Work out the finished part from the listing and answer in its coordinate system (mm). Face numbers are marked on the shaded views. A direction names the side the tool comes from. Coordinates: 2 decimals unless noted, no trailing zeros. Order: outer loops, then holes, each group sorted by start corner. A loop starts at its lowest first (then second) coordinate and runs counter-clockwise, first axis right, second up. Notation, with made-up numbers: M 77,13 L 132,13 A24 ccw 132,38 Z; hole C 19.25,69.5 d3. An arc over 180 degrees is marked long. Use a Markdown table: item, result. Add a question column.
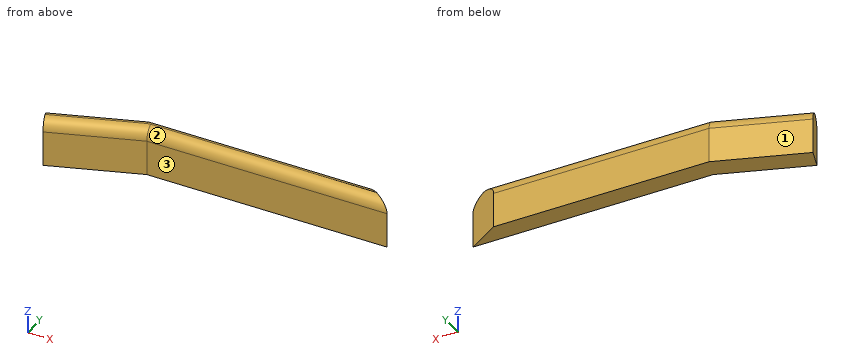
from build123d import *

# Parameters (mm, degrees)
SKETCH_1_W          = 20
SKETCH_1_H          = 4
EXTRUDE_1_DEPTH     = 1.75
EXTRUDE_2_DEPTH     = 4
EXTRUDE_3_DEPTH     = 4
CUT_EXTRUDE_1_DEPTH = 24.299797316
FILLET_4_R          = 1


with BuildPart() as part:
    # 草图1 → 凸台-拉伸1 (new body)
    with BuildSketch(Plane(origin=(0, 0, 0), x_dir=(1, 0, 0), z_dir=(0, 1, 0))):
        with Locations((10, -2)):
            Rectangle(SKETCH_1_W, SKETCH_1_H)
    extrude(amount=EXTRUDE_1_DEPTH)

    # 草图6 → 凸台-拉伸2 (add)
    with BuildSketch(Plane.XY.offset(4)):
        with BuildLine():
            Line((20, 0), (22.790216698, 0))
            ThreePointArc((22.790216698, 0), (21.391749441, 0.869644524), (20, 1.75))
            Line((20, 1.75), (20, 0))
        make_face()
    extrude(amount=-EXTRUDE_2_DEPTH)

    # 草图7 → 凸台-拉伸3 (add)
    with BuildSketch(Plane(origin=(0, 0, 0), x_dir=(-1, 0, 0), z_dir=(0, 0, -1))):
        Polygon((5.699396556, -2.736161147), (-1.818144411, 0), (-1.181196501, 1.75), (6.336344466, -0.986161147), align=None)
    extrude(amount=-EXTRUDE_3_DEPTH)

    # 草图8 → 切除-拉伸1 (cut, through all)
    with BuildSketch(Plane.XY.offset(4)):
        Polygon((1.181196501, 1.75), (-6.336344466, -0.986161147), (0, 1.75), align=None)
    extrude(amount=-CUT_EXTRUDE_1_DEPTH, mode=Mode.SUBTRACT)

    # 圆角4
    # the kernel refuses this fillet: 1 mm, written as the material it takes off along each edge
    with BuildSketch(Plane(origin=(-8.048628108, -3.591211505, 4), x_dir=(-0.3420201433256633, 0.9396926207859104, 0), z_dir=(0.9396926207859104, 0.3420201433256633, 0))) as fillet_4_piece_1_section:
        with BuildLine():
            CenterArc((FILLET_4_R, -FILLET_4_R), FILLET_4_R, 90, 90)
            Line((0, -FILLET_4_R), (0, 0))
            Line((0, 0), (FILLET_4_R, 0))
        make_face()
    fillet_4_piece_1 = extrude(amount=13, mode=Mode.PRIVATE)
    fillet_4_piece_1 = fillet_4_piece_1 - Plane(origin=(-8.048628108, 1, 3), x_dir=(0, 0, 1), z_dir=(-1, 0, 0)) * Cylinder(1, 31, mode=Mode.PRIVATE)
    add(fillet_4_piece_1, mode=Mode.SUBTRACT)
    with BuildSketch(Plane(origin=(-0.681855589, 0, 4), x_dir=(0, 1, 0), z_dir=(1, 0, 0))) as fillet_4_piece_2_section:
        with BuildLine():
            CenterArc((FILLET_4_R, -FILLET_4_R), FILLET_4_R, 90, 90)
            Line((0, -FILLET_4_R), (0, 0))
            Line((0, 0), (FILLET_4_R, 0))
        make_face()
    fillet_4_piece_2 = extrude(amount=25.972072288, mode=Mode.PRIVATE)
    fillet_4_piece_2 = fillet_4_piece_2 - Plane(origin=(-0.731431287, 0.136208109, 3), x_dir=(0, 0, 1), z_dir=(-0.9396926207859104, -0.3420201433256633, 0)) * Cylinder(1, 56, mode=Mode.PRIVATE)
    add(fillet_4_piece_2, mode=Mode.SUBTRACT)
    with BuildSketch(Plane(origin=(5.174890139, 3.203585609, 4), x_dir=(0.34202014332566305, -0.9396926207859104, 0), z_dir=(-0.9396926207859105, -0.3420201433256631, 0))) as fillet_4_piece_3:
        with BuildLine():
            CenterArc((FILLET_4_R, -FILLET_4_R), FILLET_4_R, 90, 90)
            Line((0, -FILLET_4_R), (0, 0))
            Line((0, 0), (FILLET_4_R, 0))
        make_face()
    extrude(amount=14.75, mode=Mode.SUBTRACT)
    with BuildSketch(Plane(origin=(22.5, 1.75, 4), x_dir=(0, -1, 0), z_dir=(-1, 0, 0))) as fillet_4_piece_4:
        with BuildLine():
            CenterArc((FILLET_4_R, -FILLET_4_R), FILLET_4_R, 90, 90)
            Line((0, -FILLET_4_R), (0, 0))
            Line((0, 0), (FILLET_4_R, 0))
        make_face()
    extrude(amount=25.568803499, mode=Mode.SUBTRACT)


solid = part.part
(1) A cutting plane is placed at A-A on x = 9.5. Write down the section's boundary in (y, z) (3 decimals).
(2) Which of the six approach directions +Z, -Z, +X, -X, +Y, -Y give full straight-line access (tool end or side, diameter ignored) to the marked faces 1, 2 and 3?
(3) Straight lines are drawn through the part: line 1 (Y direction, x = 18.5, z = 1.9); line 2 (Z direction, x = -2.5, y = -0.9); line 3 (Y direction, x = 1.5, z = 2.7). For each, find the intervals that lie inside material, in ascending order.
(4) A cutting plane is placed at B-B on z = 0.8. Write down the section's boundary in (x, y).
(5) Given P1, Ø2, axis at x = 2.5, z = 3.5, coming from the -Y side; P2, Ø1, axis at x = 12, z = 1.5, coming from the -Y side; P3, Ø1, axis at x = -2, z = 2, coming from the +Y side, each flat-ended and moving along its own axis, determine where each tip first touches the part or whether it passes through.
From the geometry:
| question | item | result |
|---|---|---|
| 1 | outline | M 0,0 L 1.75,0 L 1.75,3 A1 ccw 0.875,3.992 A1 ccw 0,3 Z |
| 2 | face 1 | +Z, -Z, -X, +Y |
| 2 | face 2 | +Z, +X, -Y |
| 2 | face 3 | +Z, -Z, +X, -Y |
| 3 | line 1 | y = 0 to 1.75 |
| 3 | line 2 | z = 0 to 3.93 |
| 3 | line 3 | y = -0.12 to 1.75 |
| 4 | outline | M -6.34,-0.99 L -5.7,-2.74 L 1.82,0 L 22.79,0 A214.5 cw 20,1.75 L 1.18,1.75 Z |
| 5 | P1 | stops at y = -0.08 |
| 5 | P2 | stops at y = 0 |
| 5 | P3 | stops at y = 0.77 |
